Here's how the part is built. I have some questions about the finished solid (model axes, mm). Give positions to 0.01 mm unless a question says otherwise; leave off trailing zeros. Order: outer loops, then holes, each group sorted by start corner. A loop starts at its lowest first (then second) coordinate and runs counter-clockwise, first axis right, second up.
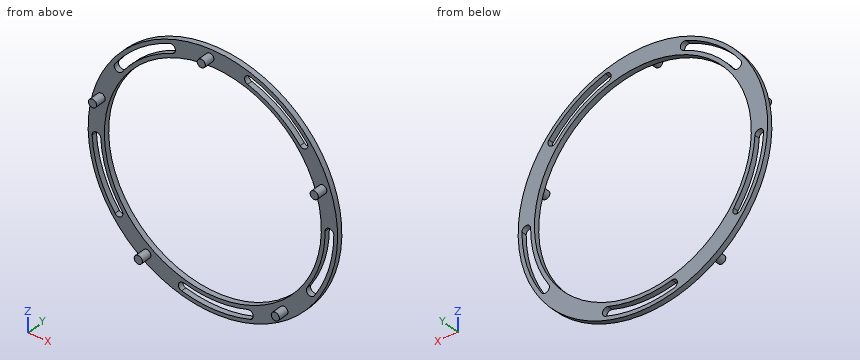
from build123d import *

# Parameters (mm, degrees)
SKETCH1_R           = 46
SKETCH1_R_2         = 40
BOSS_EXTRUDE1_DEPTH = 2
CUT_EXTRUDE1_REACH  = 67.085
SKETCH2_R           = 1.5
SKETCH3_R           = 1.5
BOSS_EXTRUDE2_DEPTH = 6
CIRPATTERN1_COUNT   = 5


with BuildPart() as part:
    # Sketch1 → Boss-Extrude1 (new body)
    with BuildSketch(Plane(origin=(0, 0, 0), x_dir=(1, 0, 0), z_dir=(0, 1, 0))):
        with Locations(Location((0, 0, 0), (0, 0, 270))):
            Circle(SKETCH1_R)
        with Locations(Location((0, 0, 0), (0, 0, 270))):
            Circle(SKETCH1_R_2, mode=Mode.SUBTRACT)
    extrude(amount=BOSS_EXTRUDE1_DEPTH)

    # Sketch2 → Cut-Extrude1 (cut, up to next)
    with BuildSketch(Plane(origin=(0, 2, 0), x_dir=(1, 0, 0), z_dir=(0, 1, 0)), mode=Mode.PRIVATE) as cut_extrude1_sk1:
        with Locations(Location((26.176741447, 34.114193633, 0), (0, 0, 270))):
            Circle(SKETCH2_R)
    cut_extrude1_tool1 = extrude(cut_extrude1_sk1.sketch, amount=-CUT_EXTRUDE1_REACH, mode=Mode.PRIVATE) & part.part
    # Sketch2 → Cut-Extrude1 (cut, up to next)
    with BuildSketch(Plane(origin=(0, 2, 0), x_dir=(1, 0, 0), z_dir=(0, 1, 0)), mode=Mode.PRIVATE) as cut_extrude1_sk2:
        with BuildLine():
            ThreePointArc((44.6, 0), (42.763360175, 12.667084374), (37.40470733, 24.290900962))
            ThreePointArc((37.40470733, 24.290900962), (35.191411966, 24.761351414), (34.720961513, 22.54805605))
            ThreePointArc((34.720961513, 22.54805605), (39.695137024, 11.758235271), (41.4, 0))
            ThreePointArc((41.4, 0), (43, -1.6), (44.6, 0))
        make_face()
    cut_extrude1_tool2 = extrude(cut_extrude1_sk2.sketch, amount=-CUT_EXTRUDE1_REACH, mode=Mode.PRIVATE) & part.part
    cut_extrude1_1 = cut_extrude1_tool1.solids().sort_by_distance((26.176741, 2, -34.114194))[0]
    add(cut_extrude1_1, mode=Mode.SUBTRACT)
    cut_extrude1_2 = cut_extrude1_tool2.solids().sort_by_distance((40.557599, 2, -12.013708))[0]
    add(cut_extrude1_2, mode=Mode.SUBTRACT)
    cut_extrude1 = cut_extrude1_1 + cut_extrude1_2  # Cut-Extrude1 as one shape, for the pattern or mirror that repeats it

    # Sketch3 → Boss-Extrude2 (add)
    with BuildSketch(Plane(origin=(0, 2, 0), x_dir=(1, 0, 0), z_dir=(0, 1, 0))):
        with Locations(Location((26.176741447, 34.114193633, 0), (0, 0, 270))):
            Circle(SKETCH3_R)
    boss_extrude2 = extrude(amount=-BOSS_EXTRUDE2_DEPTH)

    # CirPattern1: Cut-Extrude1, Boss-Extrude2 ×5 about axis
    cirpattern1_axis = Axis((0, 0, 0), (0, 1, 0))
    add([cut_extrude1.rotate(cirpattern1_axis, i * 360 / CIRPATTERN1_COUNT) for i in range(1, CIRPATTERN1_COUNT)], mode=Mode.SUBTRACT)
    add([boss_extrude2.rotate(cirpattern1_axis, i * 360 / CIRPATTERN1_COUNT) for i in range(1, CIRPATTERN1_COUNT)])


solid = part.part
Q1. I'm going to push flat-ended pins straight in: P1, Ø8, axis at x = -24, z = 31.5, coming from the -Y side; P2, Ø3, axis at x = 27.5, y = 1, coming from the -Z side. Where does each tip first touch, or does it pass through?
Filled sheet:
P1: stops at y = 0
P2: stops at z = -37.95
Q2. If we section it at A-A on z = -38: List the corners of the cut face in (x, y) for me.
Filled sheet:
outline: (-25.92, 0) - (-12.49, 0) - (-12.49, 2) - (-25.92, 2) - close; (12.49, 0) - (25.92, 0) - (25.92, 2) - (12.49, 2) - close
Q3. If we section it at D-D on z = -8.5: List the corners of the cut face in (x, y) for me, plus the area to 3 significant figures.
Filled sheet:
outline: (-45.21, 0) - (-43.78, 0) - (-43.78, 2) - (-45.21, 2) - close; (-40.52, 0) - (-39.09, 0) - (-39.09, 2) - (-40.52, 2) - close; (39.09, 0) - (40.52, 0) - (40.52, 2) - (39.09, 2) - close; (43.78, 0) - (45.21, 0) - (45.21, 2) - (43.78, 2) - close
area: 11.4 mm2
Q4. If we section it at C-C on y = -2.3: List the corners of the cut face in (x, z) for me.
Filled sheet:
outline: circle Ø3 at (-41.23, 12.21); circle Ø3 at (-24.36, -35.44); circle Ø3 at (-1.13, 42.99); circle Ø3 at (26.18, -34.11); circle Ø3 at (40.53, 14.35)
Q5. If we section it at B-B on x = 21: List the corners of the cut face in (y, z) for me, plus the area to 3 significant figures.
Filled sheet:
outline: (0, -40.93) - (2, -40.93) - (2, -34.04) - (0, -34.04) - close; (0, 34.04) - (2, 34.04) - (2, 35.68) - (0, 35.68) - close; (0, 39.35) - (2, 39.35) - (2, 40.93) - (0, 40.93) - close
area: 20.2 mm2
Q6. I need wall thicknesses on L1, parallel to X at y = 0.95, z = -6.5; L2, parallel to X at y = 0.8, z = 27; L3, parallel to Y at x = 41.5, z = 11.5. Which ranges of each line are inside material? Lowest first, please.
Filled sheet:
L1: x = -45.54 to -44.12, -40.89 to -39.47, 39.47 to 40.89, 44.12 to 45.54
L2: x = -37.24 to -35.5, -31.38 to -29.51, 29.51 to 31.38, 35.02 to 37.24
L3: y = 0 to 2
